CAD build for the part. Positions are in the model's coordinates, mm. A direction names the side the tool comes from. Give positions to 0.01 mm unless a question says otherwise; leave off trailing zeros. Order: outer loops, then holes, each group sorted by start corner. A loop starts at its lowest first (then second) coordinate and runs counter-clockwise, first axis right, second up. Notation, with made-up numbers: (79.5, 81) -> (99.5, 81) arc R33 cw to (99.5, 115) -> close; hole circle Ø3 at (9, 77.25). An arc over 180 degrees is marked (long way). Use one line per item in the form item = value. Start each with the question number.
1) Tool access for faces 4 (the face through (-6.97, 31.69, 2.54)), 5 (the face through (11, -36, 5)), 6 (the face through (-20, 31, 8.3)): list every direction of +Z, -Z, +X, -X, +Y, -Y with a clear straight run to the whole face (end or side of a thin tool).
2) Mould opens along Y. For faces 1 (the face through (0, 7, 3)), 2 (the face through (35.69, -11.24, 6.63)), 3 (the face through (-26.31, -26.61, 2.46)) say: pulls with the +Y half, pulls with the -Y half, needs draft (parallel to the pull), parting line crosses it, or undercut.
3) Drop flat-ended pins along their axis: P1, Ø2, axis at x = 9.5, z = 7.5, coming from the +Y side; P2, Ø21.5, axis at x = -7, y = 5, coming from the +Z side; P3, Ø3, axis at y = 28, z = 4.5, coming from the +X side. Give the stop position or say it passes through.
4) Cut at A-A, the plane x = 0. State how many separate pieces and enclosed holes the cut face has, and give its area (3 significant figures).
5) Cut at C-C, the plane z = 1.5. Give the cut face in (x, y).
6) Probe line 1 (Y direction, x = -1, z = 4.25); line 2 (Y direction, x = -5.5, z = 3.25); line 3 (Y direction, x = 0, z = 6). List the from-to ranges inside material, lowest first.
7) Cut at B-B, the plane y = 9. Give the cut face in (x, z), and give its area (3 significant figures).
8) Cut at D-D, the plane y = -18.5. Give the cut face in (x, z).
Autodesk Inventor part; units mm, degrees
ref_plane "YZ Plane" through (0, 0, 0) normal (1, 0, 0) x (0, 1, 0)
ref_plane "XZ Plane" through (0, 0, 0) normal (0, 1, 0) x (-1, 0, 0)
ref_plane "XY Plane" through (0, 0, 0) normal (0, 0, 1) x (1, 0, 0)
sketch "Sketch1" plane through (0, 0, 0) normal (0, 0, 1) x (1, 0, 0)
  line L0 (37.4203, -15.5) -> (15.5, -37.4203)
  line L1 (15.5, -37.4203) -> (-15.5, -37.4203)
  line L2 (-15.5, -37.4203) -> (-37.4203, -15.5)
  line L3 (-37.4203, -15.5) -> (-37.4203, 15.5)
  line L4 (-37.4203, 15.5) -> (-15.5, 37.4203)
  line L5 (-15.5, 37.4203) -> (15.5, 37.4203)
  line L6 (15.5, 37.4203) -> (37.4203, 15.5)
  line L7 (37.4203, 15.5) -> (37.4203, -15.5)
  point P0 (0, 0)
  point P1 (0, 0)
  dimension "d0" = 31
  dimension "d1" = 0
extrude "Extrusion3" add sketch "Sketch1" along normal blind 5
sketch "Sketch5" plane through (0, 0, 5) normal (0, 0, 1) x (1, 0, 0)
  circle A0 centre (0, 0) radius 36
  circle A1 centre (0, 0) radius 37.42
  line L0 (-7, 15) -> (7, 15)
  line L1 (7, 15) -> (7, 7)
  line L2 (7, 7) -> (-7, 7)
  line L3 (-7, 7) -> (-7, 15)
  line L4 (0, 29) -> (0, 22) construction
  line L5 (0, 29) -> (7, 29) construction
  circle A2 centre (0, 0) radius 29
  line L6 (-6, 28.3725) -> (-7.9667, 35.1074)
  line L7 (6, 28.3725) -> (7.9667, 35.1074)
  dimension "d14" = 72
  dimension "d15" = 74.84
  dimension "d16" = 14
  dimension "d17" = 8
  dimension "d18" = 7
  dimension "d19" = 15
  dimension "d24" = 29
  dimension "d27" = 6
  dimension "d28" = 0
extrude "Extrusion4" add sketch "Sketch5" along normal blind 3.3 contours A1
extrude "Extrusion5" cut sketch "Sketch5" against normal blind 5 contours L0 L1 L2 L3
extrude "Extrusion6" cut sketch "Sketch5" against normal blind 5 contours L7 A2 L6 A0 picked at (-0.671, 33.577)
properties part number "LEDR03"
Result:
q1.face_4 = +Z, -Z
q1.face_5 = +Z
q1.face_6 = +Z, +X, -X, +Y, -Y
q2.face_1 = undercut
q2.face_2 = parting line crosses it
q2.face_3 = pulls with the -Y half
q3.P1 = 36.44
q3.P2 = 5
q3.P3 = 26.42
q4.separate_pieces = 3
q4.enclosed_holes = 0
q4.area = 309 mm²
q5.outline = (-37.42, -15.5) -> (-15.5, -37.42) -> (15.5, -37.42) -> (37.42, -15.5) -> (37.42, 15.5) -> (15.5, 37.42) -> (-15.5, 37.42) -> (-37.42, 15.5) -> close; hole (-7.97, 35.11) -> (-6, 28.37) arc R29 cw to (6, 28.37) -> (7.97, 35.11) arc R36 ccw to start; hole (-7, 7) -> (7, 7) -> (7, 15) -> (-7, 15) -> close
q6.line_1 = -37.42 to 7, 15 to 28.98, 35.99 to 37.42
q6.line_2 = -37.42 to 7, 15 to 28.47, 35.58 to 37.42
q6.line_3 = -37.42 to -36, 36 to 37.42
q7.outline = (-37.42, 0) -> (-7, 0) -> (-7, 5) -> (-34.86, 5) -> (-34.86, 8.3) -> (-36.32, 8.3) -> (-36.32, 5) -> (-37.42, 5) -> close; (7, 0) -> (37.42, 0) -> (37.42, 5) -> (36.32, 5) -> (36.32, 8.3) -> (34.86, 8.3) -> (34.86, 5) -> (7, 5) -> close
q7.area = 314 mm²
q8.outline = (-34.42, 0) -> (34.42, 0) -> (34.42, 5) -> (32.53, 5) -> (32.53, 8.3) -> (30.88, 8.3) -> (30.88, 5) -> (-30.88, 5) -> (-30.88, 8.3) -> (-32.53, 8.3) -> (-32.53, 5) -> (-34.42, 5) -> close
